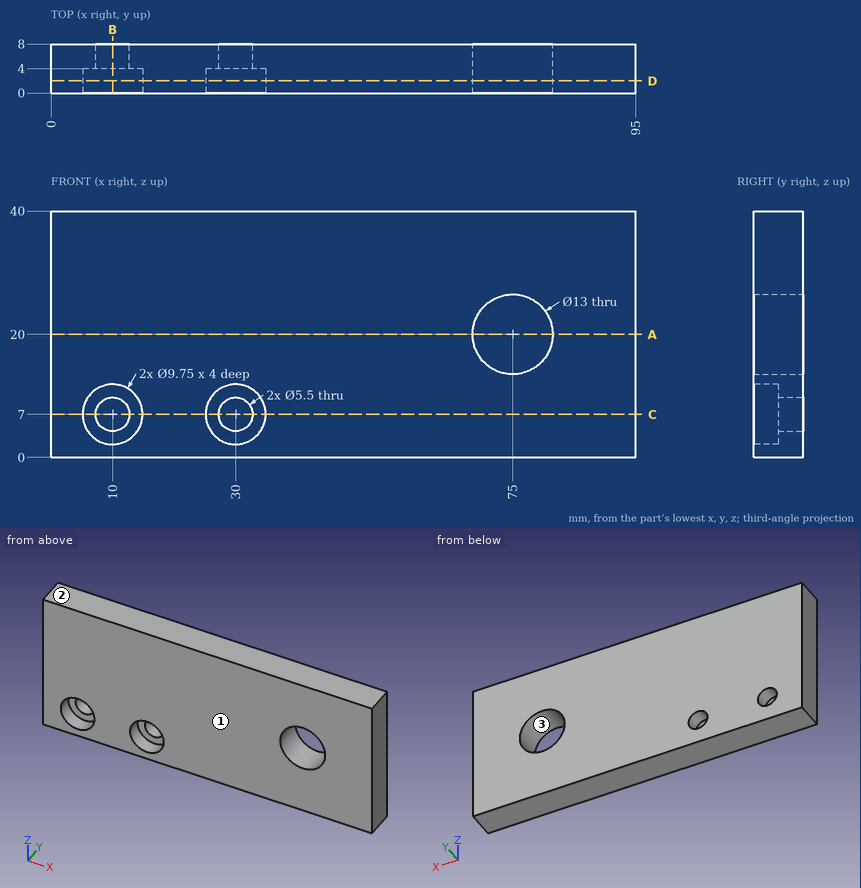
Could you check a few things on this drawing? It's one solid part, dimensions in mm from its lowest x, y, z. Give positions to 0.01 mm unless a question says otherwise; leave off trailing zeros. Write each loop counter-clockwise with the first axis right and the second up, starting at its lowest first coordinate (ties: lowest second). Pieces come first, ordered by that corner, then holes. Notation, with made-up numbers: (11, -22) -> (66, -22) arc R13 ccw to (66, -7) -> close; hole circle Ø10 at (47, 63.25). An arc over 180 degrees is marked (long way). Answer as a JSON object with one key per item and string values.
Q1. Please list where these lines run through material, in increasing order: L1, parallel to Z at x = 75, y = 5; L2, parallel to Z at x = 30, y = 4.95; L3, parallel to X at y = 0.75, z = 26.
Taken from the geometry:
{"L1": "z = 0 to 13.5, 26.5 to 40", "L2": "z = 0 to 4.25, 9.75 to 40", "L3": "x = 0 to 72.5, 77.5 to 95"}
Q2. Suppose I cut it at C-C on z = 7. Write out the boundary of the cut face in (x, y) (3 decimals), then the cut area to 3 significant figures.
Taken from the geometry:
{"outline": "(0, 0) -> (5.125, 0) -> (5.125, 4) -> (7.25, 4) -> (7.25, 8) -> (0, 8) -> close; (12.75, 4) -> (14.875, 4) -> (14.875, 0) -> (25.125, 0) -> (25.125, 4) -> (27.25, 4) -> (27.25, 8) -> (12.75, 8) -> close; (32.75, 4) -> (34.875, 4) -> (34.875, 0) -> (95, 0) -> (95, 8) -> (32.75, 8) -> close", "area": "638 mm²"}
Q3. Suppose I cut it at D-D on y = 2. Write out the boundary of the cut face in (x, z) (3 decimals).
Taken from the geometry:
{"outline": "(0, 0) -> (95, 0) -> (95, 40) -> (0, 40) -> close; hole circle Ø9.75 at (10, 7); hole circle Ø9.75 at (30, 7); hole circle Ø13 at (75, 20)"}
Q4. Suppose I cut it at B-B on x = 10. Write out the boundary of the cut face in (y, z) (3 decimals), then the cut area to 3 significant figures.
Taken from the geometry:
{"outline": "(0, 0) -> (8, 0) -> (8, 4.25) -> (4, 4.25) -> (4, 2.125) -> (0, 2.125) -> close; (0, 11.875) -> (4, 11.875) -> (4, 9.75) -> (8, 9.75) -> (8, 40) -> (0, 40) -> close", "area": "259 mm²"}
Q5. Will these pins go through, and if not, where does the flat tip stop? pin 1 Ø8 at (x, z) = (31, 5.5) entering from -Y; pin 2 Ø9 at (x, z) = (10, 7) entering from -Y.
Taken from the geometry:
{"pin 1": "stops at y = 0", "pin 2": "stops at y = 4"}
Q6. We'd pull the mould along Z, two halves only. Please class the marked faces 1, 2 and 3: released by +Z, released by -Z, zero draft, split by the parting line, or undercut.
Taken from the geometry:
{"face 1": "zero draft", "face 2": "released by +Z", "face 3": "undercut"}
Q7. Suppose I cut it at A-A on z = 20. Write out the boundary of the cut face in (x, y), then the cut area to 3 significant figures.
Taken from the geometry:
{"outline": "(0, 0) -> (68.5, 0) -> (68.5, 8) -> (0, 8) -> close; (81.5, 0) -> (95, 0) -> (95, 8) -> (81.5, 8) -> close", "area": "656 mm²"}
